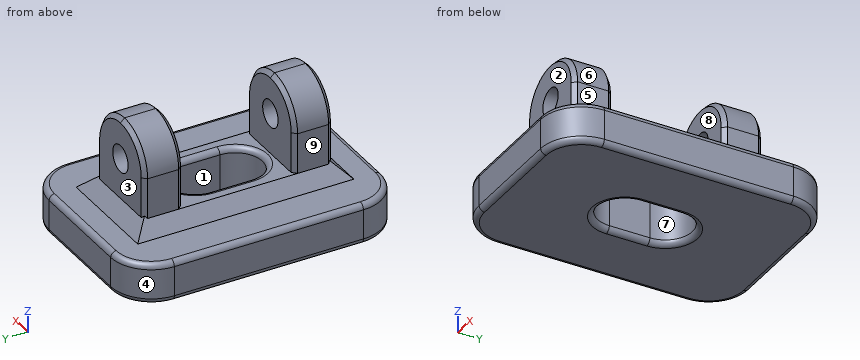
from build123d import *

# Parameters (mm, degrees)
BOSS_EXTRUDE1_DEPTH = 3
SKETCH2_W           = 6
SKETCH2_H           = 14
BOSS_EXTRUDE2_DEPTH = 1
SKETCH3_W           = 6
SKETCH3_H           = 2.9
BOSS_EXTRUDE3_DEPTH = 6
SKETCH4_R           = 1
CUT_EXTRUDE1_DEPTH  = 21.928449536
FILLET1_R           = 3
CHAMFER1_SIZE       = 1
CHAMFER2_SIZE       = 0.3
CUT_EXTRUDE2_DEPTH  = 14.601470509
FILLET2_R           = 0.4


with BuildPart() as part:
    # Sketch1 → Boss-Extrude1 (new body)
    with BuildSketch(Plane.XY):
        with BuildLine():
            Line((-4, -10), (4, -10))
            ThreePointArc((4, -10), (6.121320344, -9.121320344), (7, -7))
            Line((7, -7), (7, 7))
            ThreePointArc((7, 7), (6.121320344, 9.121320344), (4, 10))
            Line((4, 10), (-4, 10))
            ThreePointArc((-4, 10), (-6.121320344, 9.121320344), (-7, 7))
            Line((-7, 7), (-7, -7))
            ThreePointArc((-7, -7), (-6.121320344, -9.121320344), (-4, -10))
        make_face()
    extrude(amount=BOSS_EXTRUDE1_DEPTH)

    # Sketch2 → Boss-Extrude2 (add)
    with BuildSketch(Plane.XY.offset(3)):
        Rectangle(SKETCH2_W, SKETCH2_H)
    extrude(amount=BOSS_EXTRUDE2_DEPTH)

    # Sketch3 → Boss-Extrude3 (add)
    with BuildSketch(Plane.XY.offset(4)):
        with Locations((0, 5.55)):
            Rectangle(SKETCH3_W, SKETCH3_H)
        with Locations((0, -5.55)):
            Rectangle(SKETCH3_W, SKETCH3_H)
    extrude(amount=BOSS_EXTRUDE3_DEPTH)

    # Sketch4 → Cut-Extrude1 (cut, through all)
    with BuildSketch(Plane(origin=(0, 7, 0), x_dir=(1, 0, 0), z_dir=(0, 1, 0))):
        with Locations(Location((0, -7, 0), (0, 0, 90))):
            Circle(SKETCH4_R)
    extrude(amount=-CUT_EXTRUDE1_DEPTH, mode=Mode.SUBTRACT)

    # Fillet1
    fillet1_edges = [part.edges().sort_by_distance(p)[0] for p in [
        (3, -5.55, 10),
        (-3, -5.55, 10),
        (-3, 5.55, 10),
        (3, 5.55, 10),
    ]]
    fillet(fillet1_edges, radius=FILLET1_R - 0.0001)  # a hair under: the kernel refuses the full size

    # Chamfer1
    chamfer1_edges = [part.edges().sort_by_distance(p)[0] for p in [
        (3, 0, 3),
        (0, 7, 3),
        (-3, 0, 3),
        (0, -7, 3),
    ]]
    chamfer(chamfer1_edges, length=CHAMFER1_SIZE - 0.0001)  # a hair under: the kernel refuses the full size

    # Chamfer2
    chamfer2_edges = [part.edges().sort_by_distance(p)[0] for p in [
        (-3, -4.1, 5.50005),
        (3, -4.1, 5.50005),
        (-2.121349633, -4.1, 9.121349633),
        (2.121349633, -4.1, 9.121349633),
        (3, 7, 5.5),
        (3, 4.1, 5.50005),
        (3, -7, 5.5),
        (-3, -7, 5.5),
        (-2.121349633, -7, 9.121349633),
        (2.121349633, -7, 9.121349633),
        (-3, 4.1, 5.50005),
        (-3, 7, 5.5),
        (2.121349633, 4.1, 9.121349633),
        (-2.121349633, 4.1, 9.121349633),
        (2.121349633, 7, 9.121349633),
        (-2.121349633, 7, 9.121349633),
    ]]
    chamfer(chamfer2_edges, length=CHAMFER2_SIZE)

    # Sketch5 → Cut-Extrude2 (cut, through all)
    with BuildSketch(Plane.XY.offset(4)):
        with BuildLine():
            Line((-2, -1.5), (-2, 1.5))
            ThreePointArc((-2, 1.5), (0, 3.5), (2, 1.5))
            Line((2, 1.5), (2, -1.5))
            ThreePointArc((2, -1.5), (0, -3.5), (-2, -1.5))
        make_face()
    extrude(amount=-CUT_EXTRUDE2_DEPTH, mode=Mode.SUBTRACT)

    # Fillet2
    fillet2_edges = [part.edges().sort_by_distance(p)[0] for p in [
        (6.121320344, -9.121320344, 0),
        (7, 0, 0),
        (6.121320344, 9.121320344, 0),
        (0, 10, 0),
        (7, 0, 3),
        (6.121320344, -9.121320344, 3),
        (0, -3.5, 0),
        (-2, 0, 0),
        (0, 3.5, 0),
        (2, 0, 0),
        (0, -3.5, 4),
        (2, 0, 4),
        (0, 3.5, 4),
        (-2, 0, 4),
        (0, -10, 3),
        (-6.121320344, -9.121320344, 3),
        (-7, 0, 3),
        (-6.121320344, 9.121320344, 3),
        (0, 10, 3),
        (-6.121320344, 9.121320344, 0),
        (6.121320344, 9.121320344, 3),
        (-7, 0, 0),
        (-6.121320344, -9.121320344, 0),
        (0, -10, 0),
    ]]
    fillet(fillet2_edges, radius=FILLET2_R)


solid = part.part
Source: CAD feature listing. Evaluate the final solid. Frame: model axes, mm. Face numbers are marked on the shaded views. A direction names the side the tool comes from. Coordinates: 2 decimals unless noted, no trailing zeros. Loops run counter-clockwise (first coordinate to the right, second up) from the corner with the lowest first, then second, coordinate; pieces in that order, holes last. Notation, with made-up numbers: (-6, -8.5) - (32, -8.5) arc R19 cw to (32, 7.5) - close; hole circle Ø11 at (32, -3.5). An arc over 180 degrees is marked (long way). One line per item, written item: value. Start each with the question number.
1. Mould query, pull axis X, two halves, no side actions, for the marked faces 6, 7, 8 and 9. Classes: pulls with the +X half, pulls with the -X half, needs draft (parallel to the pull), parting line crosses it, or undercut.
2. Contact query for flat-ended pins moving along their axis: P1, Ø2.5, axis at x = -1.5, z = 7.5, coming from the -Y side; P2, Ø1.8, axis at x = 0, z = 7, coming from the +Y side; P3, Ø3.5, axis at y = -2.5, z = 6, coming from the +X side; P4, Ø2.5, axis at y = -2, z = 5, coming from the -X side. Output: stop coordinate, or through.
3. Set-up query: the marked faces 1, 2, 3, 4 and 5. Return all of +Z, -Z, +X, -X, +Y, -Y with unobstructed straight access to the full face (end or side cutting, diameter ignored); none if empty.
4. Section A-A (z = 4.5). Return the cut outline in (x, y), and give its area (3 significant figures).
5. Ray query, L1, parallel to X at y = 5.3, z = 7; L2, parallel to Y at x = 2, z = 6.75; L3, parallel to X at y = -2, z = 3.5. Return the intervals inside material, ascending.
6. Section B-B (x = -3.25). Return the cut outline in (y, z).
Verdict:
1. face 6: pulls with the +X half
1. face 7: undercut
1. face 8: needs draft
1. face 9: pulls with the -X half
2. P1: stops at y = -7
2. P2: passes through
2. P3: stops at x = 2.85
2. P4: stops at x = -3.25
3. face 1: +Z, -Z
3. face 2: +Z, +X, -X, -Y
3. face 3: +Z, +X, -X, +Y
3. face 4: +Z, -Z, -X, +Y
3. face 5: +Z, +X, +Y, -Y
4. outline: (-3, -6.7) - (-2.7, -7) - (2.7, -7) - (3, -6.7) - (3, -4.4) - (2.7, -4.1) - (-2.7, -4.1) - (-3, -4.4) - close; (-3, 4.4) - (-2.7, 4.1) - (2.7, 4.1) - (3, 4.4) - (3, 6.7) - (2.7, 7) - (-2.7, 7) - (-3, 6.7) - close
4. area: 34.4 mm2
5. L1: x = -3 to -1, 1 to 3
5. L2: y = -7 to -4.1, 4.1 to 7
5. L3: x = -3.5 to -1.94, 1.94 to 3.5
6. outline: (-10, 0.4) arc R0.4 ccw to (-9.6, 0) - (9.6, 0) arc R0.4 ccw to (10, 0.4) - (10, 2.6) arc R0.4 ccw to (9.6, 3) - (8, 3) - (7.25, 3.75) - (-7.25, 3.75) - (-8, 3) - (-9.6, 3) arc R0.4 ccw to (-10, 2.6) - close
